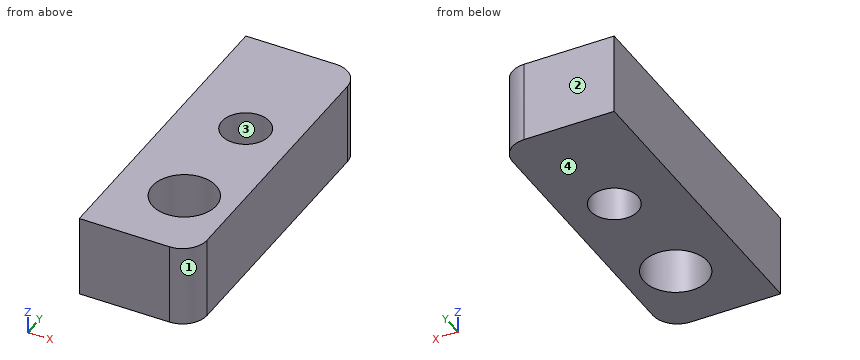
```python
from build123d import *

# Parameters (mm, degrees)
SKETCH1_R           = 1.95
SKETCH1_R_2         = 1.45
BOSS_EXTRUDE2_DEPTH = 5


with BuildPart() as part:
    # Sketch1 → Boss-Extrude2 (new body)
    with BuildSketch(Plane.XY):
        with BuildLine():
            Line((20, -9.5), (20, 9.5))
            Line((20, 9.5), (25.5, 9.5))
            ThreePointArc((25.5, 9.5), (26.560660172, 9.060660172), (27, 8))
            Line((27, 8), (27, -8))
            ThreePointArc((27, -8), (26.560660172, -9.060660172), (25.5, -9.5))
            Line((25.5, -9.5), (20, -9.5))
        make_face()
        with Locations((24, -5)):
            Circle(SKETCH1_R, mode=Mode.SUBTRACT)
        with Locations((24, 2)):
            Circle(SKETCH1_R_2, mode=Mode.SUBTRACT)
    extrude(amount=-BOSS_EXTRUDE2_DEPTH)


solid = part.part
```
Geometry check sheet. Reference: the model listing, model coordinates, mm. Face numbers are marked on the shaded views. Round coordinates to 2 decimals unless told otherwise and drop trailing zeros. Order: outer loops, then holes, each group sorted by start corner. A loop starts at its lowest first (then second) coordinate and runs counter-clockwise, first axis right, second up. Notation, with made-up numbers: (42.5, -11.75) - (68.5, -11.75) arc R32 cw to (68.5, 14.25) - close; hole circle Ø9 at (60, 77). An arc over 180 degrees is marked (long way). Use a Markdown table: item, result. Add a question column.
1) Section check A-A (y = 3). Record the cut outline in (x, z).
2) Section check C-C (z = -3.8). Record the cut outline in (x, y).
3) Mould release check, pull along Y, two halves, no side actions. Record for the marked faces 1, 2, 3 and 4: released by +Y, released by -Y, zero draft, split by the parting line, or undercut.
4) Section check B-B (x = 24). Record the cut outline in (y, z).
5) Thickness scan on line 1 along Y through (x, z) = (24, -3.9); line 2 along X through (y, z) = (3, -3.25); line 3 along Y through (x, z) = (24.75, -1.2). Record the ranges inside material, lowest first.
6) Section check D-D (y = -5). Record the cut outline in (x, z), then the cut area to 3 significant figures.
Established:
| question | item | result |
|---|---|---|
| 1 | outline | (20, -5) - (22.95, -5) - (22.95, 0) - (20, 0) - close; (25.05, -5) - (27, -5) - (27, 0) - (25.05, 0) - close |
| 2 | outline | (20, -9.5) - (25.5, -9.5) arc R1.5 ccw to (27, -8) - (27, 8) arc R1.5 ccw to (25.5, 9.5) - (20, 9.5) - close; hole circle Ø3.9 at (24, -5); hole circle Ø2.9 at (24, 2) |
| 3 | face 1 | released by -Y |
| 3 | face 2 | released by +Y |
| 3 | face 3 | undercut |
| 3 | face 4 | zero draft |
| 4 | outline | (-9.5, -5) - (-6.95, -5) - (-6.95, 0) - (-9.5, 0) - close; (-3.05, -5) - (0.55, -5) - (0.55, 0) - (-3.05, 0) - close; (3.45, -5) - (9.5, -5) - (9.5, 0) - (3.45, 0) - close |
| 5 | line 1 | -9.5 to -6.95, -3.05 to 0.55, 3.45 to 9.5 |
| 5 | line 2 | 20 to 22.95, 25.05 to 27 |
| 5 | line 3 | -9.5 to -6.8, -3.2 to 0.76, 3.24 to 9.5 |
| 6 | outline | (20, -5) - (22.05, -5) - (22.05, 0) - (20, 0) - close; (25.95, -5) - (27, -5) - (27, 0) - (25.95, 0) - close |
| 6 | area | 15.5 mm2 |
